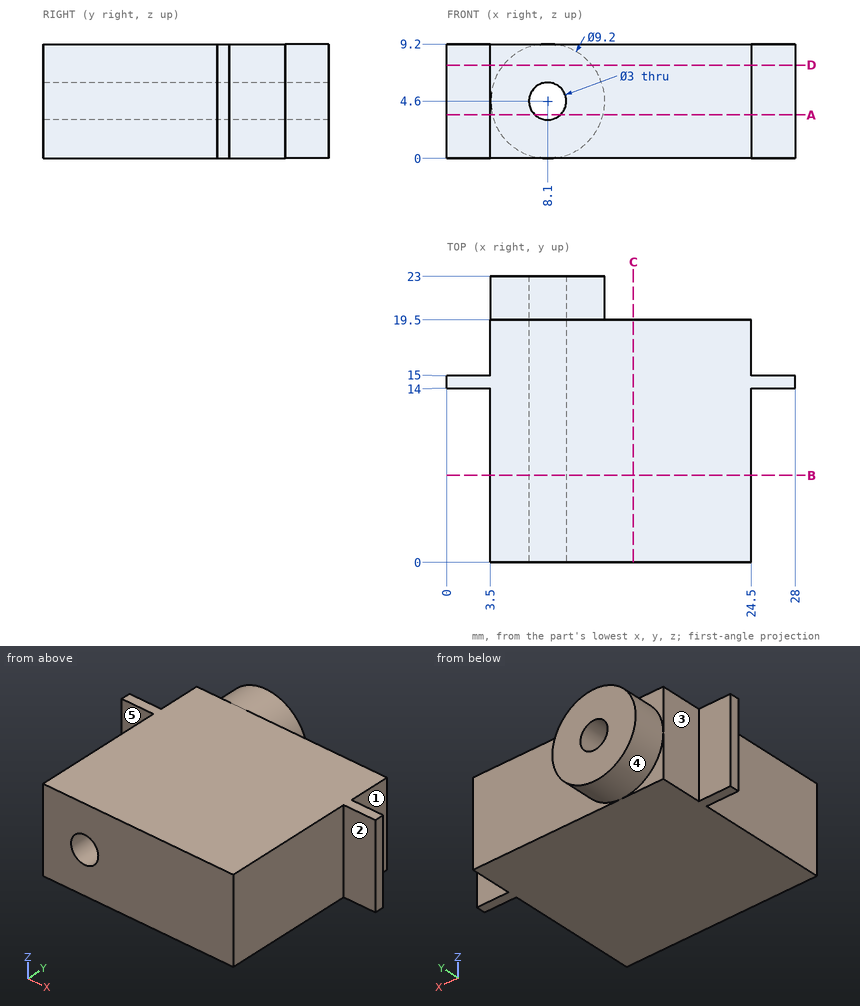
Study the drawing (mm; zero at the part's minimum x, y, z) and answer. A direction names the side the tool comes from. Round coordinates to 2 decimals unless told otherwise and drop trailing zeros. Write each loop counter-clockwise with the first axis right and the second up, starting at its lowest first coordinate (ties: lowest second). Pieces come first, ordered by that corner, then holes. Notation, with made-up numbers: (64, 50) -> (93, 50) arc R23 ccw to (93, 64) -> close; hole circle Ø10 at (-36, -36). An arc over 180 degrees is marked (long way). Answer as CSV lines item,"result". Start each with the question number.
(1) Each of these flat-tipped pins is pushed along its axis until it touches: pin 1 (3.5 mm diameter, centred on y = 18, z = 2.5, fed in from +X); pin 2 (1.8 mm diameter, centred on x = 1, z = 5, fed in from -Y); pin 3 (1.8 mm diameter, centred on x = 8.1, z = 4.6, fed in from -Y); pin 4 (1 mm diameter, centred on x = 27, z = 3.5, fed in from +Y). Where does it stop, or does it pass through?
(2) The part is cut by section B-B, the plane y = 7. Give the vertices of the cut face in (x, z).
(3) The part is cut by section C-C, the plane x = 15. Give the vertices of the cut face in (y, z).
(4) Find the intervals of material crossed by probe 1 along X at (y, z) = (11.25, 4.6); probe 2 along Z at (x, y) = (8.1, 5.25); probe 3 along Y at (x, z) = (3.25, 8.75), in increasing order.
(5) The part is cut by section A-A, the plane z = 3.5. Give the vertices of the cut face in (x, y).
(6) The part is cut by section D-D, the plane z = 7.5. Give the vertices of the cut face in (x, y), then the cut area to 3 significant figures.
(7) A tool of negligible diameter and unlimited length cuts with its end or side. For the marked faces 1, 2, 3, 4 and 5, from which of +Z, -Z, +X, -X, +Y, -Y can it reach the whole face along a straight path? Write none if from no direction.
Output values:
1,pin 1,"stops at x = 24.5"
1,pin 2,"stops at y = 14"
1,pin 3,"passes through"
1,pin 4,"stops at y = 15"
2,outline,"(3.5, 0) -> (24.5, 0) -> (24.5, 9.2) -> (3.5, 9.2) -> close; hole circle Ø3 at (8.1, 4.6)"
3,outline,"(0, 0) -> (19.5, 0) -> (19.5, 9.2) -> (0, 9.2) -> close"
4,probe 1,"x = 3.5 to 6.6, 9.6 to 24.5"
4,probe 2,"z = 0 to 3.1, 6.1 to 9.2"
4,probe 3,"y = 14 to 15"
5,outline,"(0, 14) -> (3.5, 14) -> (3.5, 0) -> (7.08, 0) -> (7.08, 23) -> (3.63, 23) -> (3.63, 19.5) -> (3.5, 19.5) -> (3.5, 15) -> (0, 15) -> close; (9.12, 0) -> (24.5, 0) -> (24.5, 14) -> (28, 14) -> (28, 15) -> (24.5, 15) -> (24.5, 19.5) -> (12.57, 19.5) -> (12.57, 23) -> (9.12, 23) -> close"
6,outline,"(0, 14) -> (3.5, 14) -> (3.5, 0) -> (24.5, 0) -> (24.5, 14) -> (28, 14) -> (28, 15) -> (24.5, 15) -> (24.5, 19.5) -> (11.67, 19.5) -> (11.67, 23) -> (4.53, 23) -> (4.53, 19.5) -> (3.5, 19.5) -> (3.5, 15) -> (0, 15) -> close"
6,area,"441 mm²"
7,face 1,"+Z, -Z, +X, +Y"
7,face 2,"+Z, -Z, +X, -Y"
7,face 3,"+Z, -Z, -X, +Y"
7,face 4,"+Y"
7,face 5,"+Z, -Z, -X, -Y"
